Design review of the part built by this model. Coordinates are the model's own, in mm. Face numbers are marked on the shaded views. A direction names the side the tool comes from. Give positions to 0.01 mm unless a question says otherwise; leave off trailing zeros. Order: outer loops, then holes, each group sorted by start corner. A loop starts at its lowest first (then second) coordinate and runs counter-clockwise, first axis right, second up.
```python
from build123d import *

# Parameters (mm, degrees)
SKETCH_1_W                       = 44
SKETCH_1_H                       = 65
SM_BASE_FLANGE_1_DEPTH           = 2
SM_EDGE_FLANGE_1_STRIP_W         = 9.4732
SM_EDGE_FLANGE_1_STRIP_H         = 2
SM_EDGE_FLANGE_1_STRIP_CUT_DEPTH = 65
SM_EDGE_FLANGE_1_DEPTH           = 65
SM_EDGE_FLANGE_2_STRIP_W         = 9.4732
SM_EDGE_FLANGE_2_STRIP_H         = 2
SM_EDGE_FLANGE_2_STRIP_CUT_DEPTH = 65
SM_EDGE_FLANGE_2_DEPTH           = 65
CUT_EXTRUDE_1_DEPTH              = 2
CUT_EXTRUDE_2_DEPTH              = 2
CUT_EXTRUDE_3_DEPTH              = 2
SKETCH_16_R                      = 1
SKETCH_16_R_2                    = 4.5
SKETCH_16_R_3                    = 1.5
CUT_EXTRUDE_5_DEPTH              = 50
FILLET_2_R                       = 0.2
FILLET_3_R                       = 0.2
FILLET_4_R                       = 0.2
FILLET_5_R                       = 0.2
FILLET_7_R                       = 1


# Sheet-metal steps are written as plain solids
with BuildPart() as part:
    # Sketch 1 → 基体-法兰1 (new body)
    with BuildSketch(Plane.XY):
        with Locations((-2.910505837, -3.223735409)):
            Rectangle(SKETCH_1_W, SKETCH_1_H)
    extrude(amount=-SM_BASE_FLANGE_1_DEPTH)

    # 边线-法兰1 strip (across the edge) → 边线-法兰1 strip cut (cut)
    with BuildSketch(Plane(origin=(-24.910505837, 29.276264591, 0), x_dir=(1, 0, 0), z_dir=(0, -1, 0))):
        with Locations((-2, -1)):
            Rectangle(SM_EDGE_FLANGE_1_STRIP_W, SM_EDGE_FLANGE_1_STRIP_H)
    extrude(amount=SM_EDGE_FLANGE_1_STRIP_CUT_DEPTH, mode=Mode.SUBTRACT)

    # 边线-法兰1 section (across the edge) → 边线-法兰1 (add)
    with BuildSketch(Plane(origin=(-24.910505837, 29.276264591, 0), x_dir=(1, 0, 0), z_dir=(0, -1, 0))):
        with BuildLine():
            Line((0, 0.7366), (0, 20))
            Line((0, 20), (2, 20))
            Line((2, 20), (2, 0.7366))
            ThreePointArc((2, 0.7366), (2.215745145, 0.215745145), (2.7366, 0))
            Line((2.7366, 0), (2.7366, -2))
            ThreePointArc((2.7366, -2), (0.801531583, -1.198468417), (0, 0.7366))
        make_face()
    extrude(amount=SM_EDGE_FLANGE_1_DEPTH)

    # 边线-法兰2 strip (across the edge) → 边线-法兰2 strip cut (cut)
    with BuildSketch(Plane(origin=(19.089494163, -35.723735409, 0), x_dir=(-1, 0, 0), z_dir=(0, 1, 0))):
        with Locations((-2, -1)):
            Rectangle(SM_EDGE_FLANGE_2_STRIP_W, SM_EDGE_FLANGE_2_STRIP_H)
    extrude(amount=SM_EDGE_FLANGE_2_STRIP_CUT_DEPTH, mode=Mode.SUBTRACT)

    # 边线-法兰2 section (across the edge) → 边线-法兰2 (add)
    with BuildSketch(Plane(origin=(19.089494163, -35.723735409, 0), x_dir=(-1, 0, 0), z_dir=(0, 1, 0))):
        with BuildLine():
            Line((0, 0.7366), (0, 20))
            Line((0, 20), (2, 20))
            Line((2, 20), (2, 0.7366))
            ThreePointArc((2, 0.7366), (2.215745145, 0.215745145), (2.7366, 0))
            Line((2.7366, 0), (2.7366, -2))
            ThreePointArc((2.7366, -2), (0.801531583, -1.198468417), (0, 0.7366))
        make_face()
    extrude(amount=SM_EDGE_FLANGE_2_DEPTH)

    # 草图12 → 切除-拉伸1 (cut)
    with BuildSketch(Plane(origin=(0, 0, -2), x_dir=(-1, 0, 0), z_dir=(0, 0, -1))):
        Polygon((-14.352894163, -3.223735409), (0.082078712, -0.395308284), (2.910505837, 9.276264591), (5.738932961, -0.395308284), (20.173905837, -3.223735409), (5.738932961, -6.052162533), (2.910505837, -15.723735409), (0.082078712, -6.052162533), align=None)
    extrude(amount=-CUT_EXTRUDE_1_DEPTH, mode=Mode.SUBTRACT)

    # 草图13 → 切除-拉伸2 (cut)
    with BuildSketch(Plane(origin=(0, 0, -2), x_dir=(-1, 0, 0), z_dir=(0, 0, -1))):
        with BuildLine():
            Line((2.910505837, 29.276264591), (17.910505837, 29.276264591))
            add(Edge.make_bspline(
                [(-12.089494163, 29.276264591), (2.910505837, 23.276264591), (17.910505837, 29.276264591)],
                knots=[0, 0, 0, 1, 1, 1], degree=2))
            Line((-12.089494163, 29.276264591), (2.910505837, 29.276264591))
        make_face()
    extrude(amount=-CUT_EXTRUDE_2_DEPTH, mode=Mode.SUBTRACT)

    # 草图14 → 切除-拉伸3 (cut)
    with BuildSketch(Plane(origin=(0, 0, -2), x_dir=(-1, 0, 0), z_dir=(0, 0, -1))):
        with BuildLine():
            Line((2.910505837, -35.723735409), (17.910505837, -35.723735409))
            add(Edge.make_bspline(
                [(-12.089494163, -35.723735409), (2.910505837, -29.723735409), (17.910505837, -35.723735409)],
                knots=[0, 0, 0, 1, 1, 1], degree=2))
            Line((-12.089494163, -35.723735409), (2.910505837, -35.723735409))
        make_face()
    extrude(amount=-CUT_EXTRUDE_3_DEPTH, mode=Mode.SUBTRACT)

    # 草图16 → 切除-拉伸5 (cut)
    with BuildSketch(Plane(origin=(19.089494163, 0, 0), x_dir=(0, 0, -1), z_dir=(1, 0, 0))):
        with Locations((-17.5, 26.95590493)):
            Circle(SKETCH_16_R)
        with Locations((-2.5, 26.95590493)):
            Circle(SKETCH_16_R)
        with Locations((-2.5, 11.95590493)):
            Circle(SKETCH_16_R)
        with Locations((-17.5, 11.95590493)):
            Circle(SKETCH_16_R)
        with Locations((-3, 19.45590493)):
            Circle(SKETCH_16_R)
        with Locations(Location((-17, 19.45590493, 0), (0, 0, 180))):
            Circle(SKETCH_16_R)
        with Locations((-10, 12.45590493)):
            Circle(SKETCH_16_R)
        with Locations(Location((-10, -18.903375747, 0), (0, 0, 180))):
            Circle(SKETCH_16_R)
        with Locations((-17, -25.903375747)):
            Circle(SKETCH_16_R)
        with Locations(Location((-3, -25.903375747, 0), (0, 0, 180))):
            Circle(SKETCH_16_R)
        with Locations(Location((-17.5, -18.403375747, 0), (0, 0, 180))):
            Circle(SKETCH_16_R)
        with Locations(Location((-2.5, -18.403375747, 0), (0, 0, 180))):
            Circle(SKETCH_16_R)
        with Locations(Location((-2.5, -33.403375747, 0), (0, 0, 180))):
            Circle(SKETCH_16_R)
        with Locations(Location((-17.5, -33.403375747, 0), (0, 0, 180))):
            Circle(SKETCH_16_R)
        with Locations((-10, -3.223735409)):
            Circle(SKETCH_16_R_2)
        with Locations((-10, 5.276264591)):
            Circle(SKETCH_16_R_3)
        with Locations(Location((-10, -11.723735409, 0), (0, 0, 180))):
            Circle(SKETCH_16_R_3)
    extrude(amount=-CUT_EXTRUDE_5_DEPTH, mode=Mode.SUBTRACT)

    # 圆角2
    fillet_2_edges = [part.edges().sort_by_distance(p)[0] for p in [
        (-2.910505837, 9.276264591, -1),
    ]]
    fillet(fillet_2_edges, radius=FILLET_2_R)

    # 圆角3
    fillet_3_edges = [part.edges().sort_by_distance(p)[0] for p in [
        (-20.173905837, -3.223735409, -1),
    ]]
    fillet(fillet_3_edges, radius=FILLET_3_R)

    # 圆角4
    fillet_4_edges = [part.edges().sort_by_distance(p)[0] for p in [
        (-2.910505837, -15.723735409, -1),
    ]]
    fillet(fillet_4_edges, radius=FILLET_4_R)

    # 圆角5
    fillet_5_edges = [part.edges().sort_by_distance(p)[0] for p in [
        (14.352894163, -3.223735409, -1),
    ]]
    fillet(fillet_5_edges, radius=FILLET_5_R)

    # 圆角7
    fillet_7_edges = [part.edges().sort_by_distance(p)[0] for p in [
        (-0.082078712, -0.395308284, -1),
        (-5.738932961, -0.395308284, -1),
        (-5.738932961, -6.052162533, -1),
        (-0.082078712, -6.052162533, -1),
    ]]
    fillet(fillet_7_edges, radius=FILLET_7_R)


solid = part.part
```
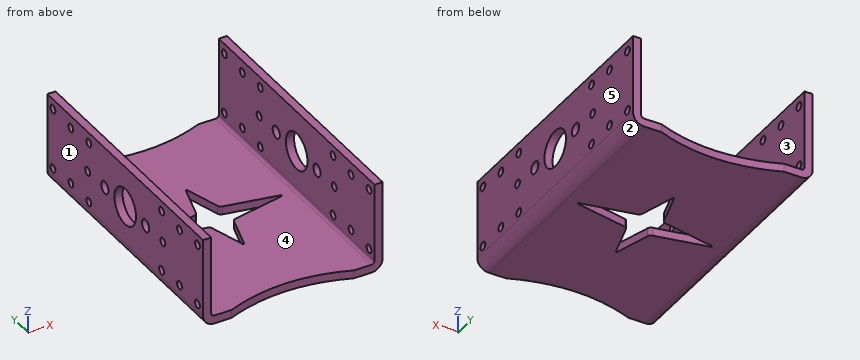
1. Take a section at B-B (y = -29). State the section outline as (x, z) points, then the cut area to 3 significant figures.
Recorded:
outline: (-24.91, 0.74) arc R2.74 ccw to (-22.17, -2) - (16.35, -2) arc R2.74 ccw to (19.09, 0.74) - (19.09, 20) - (17.09, 20) - (17.09, 0.74) arc R0.74 cw to (16.35, 0) - (-22.17, 0) arc R0.74 cw to (-22.91, 0.74) - (-22.91, 20) - (-24.91, 20) - close
area: 165 mm2
2. For pin 1 (1.6 mm diameter, centred on y = -18.9, z = 10, fed in from -X); pin 2 (6 mm diameter, centred on x = 2.5, y = 20, fed in from +Z); pin 3 (10 mm diameter, centred on x = -5, z = 1, fed in from +Y), all flat-tipped, find the tip position at first contact; note any pin that passes through.
Recorded:
pin 1: passes through
pin 2: stops at z = 0
pin 3: stops at y = 26.93
3. Take a section at C-C (x = -21.5). State the section outline as (y, z) points.
Recorded:
outline: (-35.72, -2) - (29.28, -2) - (29.28, 0) - (-35.72, 0) - close
4. For line 1 along X through (y, z) = (11.5, 8.25); line 2 along Z through (x, y) = (3, -27.5); line 3 along Y through (x, z) = (0, -1), list the stretches that pass through material, from the lowest coordinate up.
Recorded:
line 1: x = -24.91 to -22.91, 17.09 to 19.09
line 2: z = -2 to 0
line 3: y = -32.84 to -6.21, -0.24 to 26.39
5. Draft analysis for pull direction X (two halves, no side actions). For the marked faces 1, 2 and 3, state which applies: pulls with the +X half, pulls with the -X half, needs draft (parallel to the pull), parting line crosses it, or undercut.
Recorded:
face 1: pulls with the -X half
face 2: pulls with the +X half
face 3: undercut
6. Machinability: for the marked faces 4 and 5, which of the approach directions +Z, -Z, +X, -X, +Y, -Y give a long, thin tool a straight path to every point of the face, cutting with its end or side? Answer none if there is none.
Recorded:
face 4: +Z, +Y, -Y
face 5: +Z, -Z, +X, +Y, -Y
7. Take a section at A-A (y = 2). State the section outline as (x, z) points.
Recorded:
outline: (-24.91, 0.74) arc R2.74 ccw to (-22.17, -2) - (-5.04, -2) - (-5.04, 0) - (-22.17, 0) arc R0.74 cw to (-22.91, 0.74) - (-22.91, 20) - (-24.91, 20) - close; (-0.78, -2) - (16.35, -2) arc R2.74 ccw to (19.09, 0.74) - (19.09, 20) - (17.09, 20) - (17.09, 0.74) arc R0.74 cw to (16.35, 0) - (-0.78, 0) - close
